Work out the finished part from the listing and answer in its coordinate system (mm). A direction names the side the tool comes from. Round coordinates to 2 decimals unless told otherwise and drop trailing zeros. Order: outer loops, then holes, each group sorted by start corner. A loop starts at its lowest first (then second) coordinate and runs counter-clockwise, first axis right, second up. Notation, with made-up numbers: (-13, 36.5) - (25, 36.5) arc R26 cw to (25, 50.5) - close; hole circle Ø2 at (54.5, -26.5). An arc over 180 degrees is marked (long way). Use CSV: the item, a comma, the result in double quotes.
from build123d import *

# Parameters (mm, degrees)
SKETCH2_R           = 4.15
SKETCH2_R_2         = 3.96875
BOSS_EXTRUDE1_DEPTH = 15
SKETCH3_R           = 2.25
BOSS_EXTRUDE2_DEPTH = 2.25
CHAMFER1_SIZE       = 1.5
SKETCH5_R           = 20
SKETCH5_R_2         = 3.96875
BOSS_EXTRUDE4_DEPTH = 10
CHAMFER2_SIZE       = 4
CHAMFER3_SIZE       = 4


with BuildPart() as part:
    # Sketch2 → Boss-Extrude1 (new body)
    with BuildSketch(Plane.XY):
        with BuildLine():
            Line((70, 27.5), (0, 27.5))
            ThreePointArc((0, 27.5), (-27.5, 0), (0, -27.5))
            Line((0, -27.5), (70, -27.5))
            ThreePointArc((70, -27.5), (97.5, 0), (70, 27.5))
        make_face()
        Circle(SKETCH2_R, mode=Mode.SUBTRACT)
        with Locations((70, 0)):
            Circle(SKETCH2_R_2, mode=Mode.SUBTRACT)
    extrude(amount=BOSS_EXTRUDE1_DEPTH)

    # Sketch3 → Boss-Extrude2 (add)
    with BuildSketch(Plane(origin=(0, 0, 0), x_dir=(-1, 0, 0), z_dir=(0, 0, -1))):
        with Locations((-18, 0)):
            Circle(SKETCH3_R)
        with Locations((-16.217439622, 7.809907304)):
            Circle(SKETCH3_R)
        with Locations((-11.222816433, 14.072966684)):
            Circle(SKETCH3_R)
        with Locations((-4.005376811, 17.548702419)):
            Circle(SKETCH3_R)
        with Locations((4.005376811, 17.548702419)):
            Circle(SKETCH3_R)
        with Locations((11.222816433, 14.072966684)):
            Circle(SKETCH3_R)
        with Locations((16.217439622, 7.809907304)):
            Circle(SKETCH3_R)
        with Locations((18, 0)):
            Circle(SKETCH3_R)
        with Locations((16.217439622, -7.809907304)):
            Circle(SKETCH3_R)
        with Locations((11.222816433, -14.072966684)):
            Circle(SKETCH3_R)
        with Locations((4.005376811, -17.548702419)):
            Circle(SKETCH3_R)
        with Locations((-4.005376811, -17.548702419)):
            Circle(SKETCH3_R)
        with Locations((-11.222816433, -14.072966684)):
            Circle(SKETCH3_R)
        with Locations((-16.217439622, -7.809907304)):
            Circle(SKETCH3_R)
    extrude(amount=BOSS_EXTRUDE2_DEPTH)

    # Chamfer1
    chamfer1_edges = [part.edges().sort_by_distance(p)[0] for p in [
        (18.467439622, 7.809907304, -2.25),
        (13.472816433, 14.072966684, -2.25),
        (6.255376811, 17.548702419, -2.25),
        (-1.755376811, 17.548702419, -2.25),
        (-8.972816433, 14.072966684, -2.25),
        (-13.967439622, 7.809907304, -2.25),
        (-15.75, 0, -2.25),
        (-13.967439622, -7.809907304, -2.25),
        (-8.972816433, -14.072966684, -2.25),
        (-1.755376811, -17.548702419, -2.25),
        (6.255376811, -17.548702419, -2.25),
        (13.472816433, -14.072966684, -2.25),
        (18.467439622, -7.809907304, -2.25),
        (20.25, 0, -2.25),
    ]]
    chamfer(chamfer1_edges, length=CHAMFER1_SIZE)

    # Sketch5 → Boss-Extrude4 (add)
    with BuildSketch(Plane(origin=(0, 0, 0), x_dir=(-1, 0, 0), z_dir=(0, 0, -1))):
        with Locations((-70, 0)):
            Circle(SKETCH5_R)
        with Locations((-70, 0)):
            Circle(SKETCH5_R_2, mode=Mode.SUBTRACT)
    extrude(amount=BOSS_EXTRUDE4_DEPTH)

    # Chamfer2
    chamfer2_edges = [part.edges().sort_by_distance(p)[0] for p in [
        (90, 0, -10),
    ]]
    chamfer(chamfer2_edges, length=CHAMFER2_SIZE)

    # Chamfer3
    chamfer3_edges = [part.edges().sort_by_distance(p)[0] for p in [
        (-27.5, 0, 15),
        (35, -27.5, 15),
        (97.5, 0, 15),
        (35, -27.5, 0),
        (-27.5, 0, 0),
        (35, 27.5, 0),
        (97.5, 0, 0),
        (35, 27.5, 15),
    ]]
    chamfer(chamfer3_edges, length=CHAMFER3_SIZE)


solid = part.part
(1) Find section A-A (x = 31). Determine the outline of the cut face in (y, z), and give its area (3 significant figures).
Findings below:
outline,"(-27.5, 4) - (-23.5, 0) - (23.5, 0) - (27.5, 4) - (27.5, 11) - (23.5, 15) - (-23.5, 15) - (-27.5, 11) - close"
area,"793 mm²"
(2) Find the intervals of material crossed by L1, parallel to Z at x = -16, y = -5; L2, parallel to Y at x = 0, z = 9.5; L3, parallel to Y at x = 70, z = 8.25, in increasing order. Write a range as from..to.
Findings below:
L1,"z = 0..15"
L2,"y = -27.5..-4.15, 4.15..27.5"
L3,"y = -27.5..-3.97, 3.97..27.5"
(3) For faces 4 (the flat face through (34.5, -25.5, 2)), 5 (the cylindrical face through (18, 6.44, -0.37)), determine the directions among +Z, -Z, +X, -X, +Y, -Y from which every point of the face is accessible in a straight line to the end or side of a thin tool.
Findings below:
face 4,"-Z, +X, -X, -Y"
face 5,"-Z"
(4) Each of these flat-tipped pins is pushed along its axis until it touches: pin 1 (12 mm diameter, centred on y = -7, z = 11.5, fed in from -X); pin 2 (6 mm diameter, centred on x = 44.5, y = -4, fed in from -Z); pin 3 (0.8 mm diameter, centred on x = 4, y = -18, fed in from -Z). Where does it stop, or does it pass through?
Findings below:
pin 1,"stops at x = -27.48"
pin 2,"stops at z = 0"
pin 3,"stops at z = -2.25"
(5) Find section B-B (z = 8.5). Determine the outline of the cut face in (x, y).
Findings below:
outline,"(0, -27.5) - (70, -27.5) arc R27.5 ccw to (70, 27.5) - (0, 27.5) arc R27.5 ccw to start; hole circle Ø8.3 at (0, 0); hole circle Ø7.94 at (70, 0)"
(6) Find section C-C (z = -4.5). Determine the outline of the cut face in (x, y).
Findings below:
outline,"circle Ø40 at (70, 0); hole circle Ø7.94 at (70, 0)"
(7) The mould has two halves that part along X. Classify faces 1 (the flat face through (67, -3, -10)), 2 (the conical face through (93.688, -0.521, 14.806)), 3 (the cylindrical face through (2.8, 19.45, -0.37)): released by +X, released by -X, zero draft, split by the parting line, or undercut.
Findings below:
face 1,"zero draft"
face 2,"released by +X"
face 3,"undercut"
